```python
from build123d import *

# Parameters (mm, degrees)
BOSS_EXTRUDE1_DEPTH = 0.889
LOFT2_DEPTH         = 82.529690579
LOFT2_START         = 4.746357977
LOFT2_2_DEPTH       = 59.253642023
LOFT2_START_2       = -13.360997113
LOFT2_3_DEPTH       = 13.360997113
LOFT2_START_3       = -53.387286303
LOFT2_4_DEPTH       = 59.387286303
LOFT2_START_4       = -71.244406959
LOFT2_5_DEPTH       = 13.360997113


with BuildPart() as part:
    # Sketch2 → Boss-Extrude1 (new body)
    with BuildSketch(Plane.XY):
        Polygon((1.079234415, 1.079234415), (1.079234415, 81.450456164), (9.69091533, 81.450456164), (36.503516987, 71.395730542), (36.503516987, 11.133960037), (9.69091533, 1.079234415), align=None)
        Polygon((1.904531321, 1.904531321), (1.904531321, 80.625159258), (9.54126046, 80.625159258), (35.678220081, 70.8237994), (35.678220081, 11.705891179), (9.54126046, 1.904531321), align=None, mode=Mode.SUBTRACT)
    extrude(amount=BOSS_EXTRUDE1_DEPTH)

    # Loft2: read off the stored shape, not the designer's step
    # Loft2 outline → Loft2 (add)
    with BuildSketch(Plane(origin=(0, 0, 0), x_dir=(1, 0, 0), z_dir=(0, 1, 0))):
        Polygon((0, 0), (37.582751402, 0), (28.057751402, 19.05), (0, 19.05), align=None)
    extrude(amount=LOFT2_DEPTH)

    # Loft2 2 outline → Loft2 2 (cut)
    with BuildSketch(Plane(origin=(0, 0, 0), x_dir=(0.9918794395900915, -0.08993102167340751, -0.08993102167340765), z_dir=(0.12718167052860177, 0.7013646778536657, 0.7013646778536667)).offset(LOFT2_START)):
        Polygon((2.384353581, 58.357303857), (30.789607102, 51.013257415), (37, 49.40758916), (37, 73), (-9, 73), (-9, 58.357303857), align=None)
    extrude(amount=LOFT2_2_DEPTH, mode=Mode.SUBTRACT)

    # Loft2 3 outline → Loft2 3 (cut)
    with BuildSketch(Plane(origin=(0, 0, 0), x_dir=(0.9918794395900915, -0.08993102167340751, -0.08993102167340765), z_dir=(0.12718167052860177, 0.7013646778536657, 0.7013646778536667)).offset(LOFT2_START_2)):
        Polygon((37, 49.40758916), (30.789607102, 51.013257415), (2.384353581, 58.357303857), (-9, 58.357303857), (-9, 1), (37, 1), align=None)
    extrude(amount=LOFT2_3_DEPTH, mode=Mode.SUBTRACT)

    # Loft2 4 outline → Loft2 4 (cut)
    with BuildSketch(Plane(origin=(0, 0, 0), x_dir=(0.9918794395900911, 0.08993102167341009, -0.08993102167341009), z_dir=(0.12718167052860532, -0.7013646778536659, 0.7013646778536659)).offset(LOFT2_START_3)):
        Polygon((38.211586494, 7.344046443), (9.806332973, 0), (-1, 0), (-1, -15), (45, -15), (45, 9.099159244), align=None)
    extrude(amount=LOFT2_4_DEPTH, mode=Mode.SUBTRACT)

    # Loft2 5 outline → Loft2 5 (cut)
    with BuildSketch(Plane(origin=(0, 0, 0), x_dir=(0.9918794395900911, 0.08993102167341009, -0.08993102167341009), z_dir=(0.12718167052860532, -0.7013646778536659, 0.7013646778536659)).offset(LOFT2_START_4)):
        Polygon((-1, 0), (9.806332973, 0), (38.211586494, 7.344046443), (45, 9.099159244), (45, 58), (-1, 58), align=None)
    extrude(amount=LOFT2_5_DEPTH, mode=Mode.SUBTRACT)

    # Sketch5 → section 0 of cut_loft2
    with BuildSketch(Plane.XY.offset(-17.145), mode=Mode.PRIVATE) as cut_loft2_s0:
        with BuildLine():
            Line((27.105251402, 26.8023965), (6.432194068, 19.05))
            Line((6.432194068, 19.05), (1.905, 19.05))
            Line((1.905, 19.05), (1.905, 63.479690579))
            Line((1.905, 63.479690579), (6.432194068, 63.479690579))
            Line((6.432194068, 63.479690579), (27.105251402, 55.727294079))
            Line((27.105251402, 55.727294079), (27.105251402, 26.8023965))
        make_face()
    # loft up to a face of the part (cut_loft2)
    loft([cut_loft2_s0.sketch, part.faces().sort_by_distance((17.91973196, 41.264845289, 0))[0]], mode=Mode.SUBTRACT)


solid = part.part
```
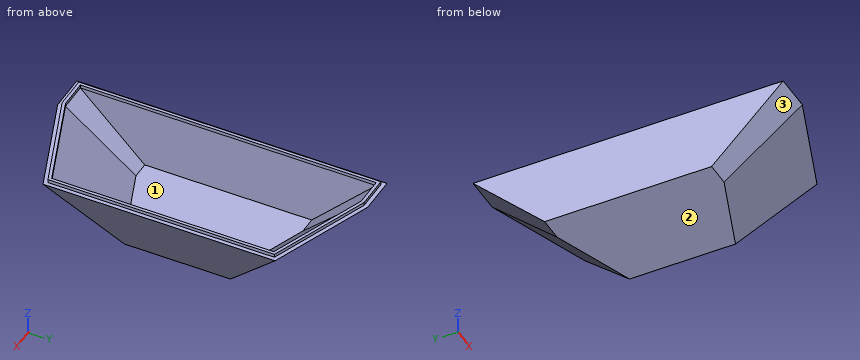
For this review, take the finished solid that the model builds, in its own axes (mm). Face numbers are marked on the shaded views. Round coordinates to 2 decimals unless told otherwise and drop trailing zeros.
(1) Wall thickness on line 1 along Z through (x, y) = (5, 40.5) (3 decimals); line 2 along Y through (x, z) = (20.5, -12.25); line 3 along Y through (x, z) = (5, -7.75): over which ranges is each line inside the solid? List them lowest first.
Returned:
line 1: z = -19.05 to -17.145
line 2: y = 17.06 to 19.1, 63.43 to 65.47
line 3: y = 7.75 to 9.65, 72.87 to 74.78
(2) Mouldability with a two-part tool opening along Y and no side actions: class the marked faces 1, 2 and 3 as released by +Y, released by -Y, zero draft, split by the parting line, or undercut.
Returned:
face 1: undercut
face 2: zero draft
face 3: released by -Y
(3) Clearance check with flat-ended pins moving along their axes: P1, Ø6, axis at y = 14, z = -12, coming from the -X side; P2, Ø11.5, axis at x = 17, y = 41, coming from the +Z side (3 decimals); P3, Ø8, axis at x = 28.5, y = 23.5, coming from the +Z side; P4, Ø5, axis at x = 14.5, y = 12.5, coming from the +Z side. State where each tip first meets the part, or that it passes through.
Returned:
P1: stops at x = 0
P2: stops at z = -17.145
P3: stops at z = -6.36
P4: stops at z = -5.68
